Part model, mm, in its own coordinate system. A direction names the side the tool comes from. Round coordinates to 2 decimals unless told otherwise and drop trailing zeros. Write each loop counter-clockwise with the first axis right and the second up, starting at its lowest first coordinate (ties: lowest second). Pieces come first, ordered by that corner, then holes.
from build123d import *

# Parameters (mm, degrees)
F0_W     = 76.4351114631
F0_H     = 77.7774527669
F1_DEPTH = 50.8
F3_DEPTH = 77.7784527669
F4_R     = 7.4764365624
F5_DEPTH = 58.8116741145
F6_W     = 82.7689305879
F6_H     = 70.0802728534
F7_DEPTH = 12.7
F9_DEPTH = 90.4784527669


with BuildPart() as f1:
    # F0 (on Top) → F1 (new body)
    with BuildSketch(Plane.XY):
        with Locations((-38.2175557315, -38.8887263834)):
            Rectangle(F0_W, F0_H)
    extrude(amount=F1_DEPTH)

    # F2 (on face) → F3 (cut, through all)
    with BuildSketch(Plane.XZ.offset(77.7774527669)):
        Polygon((15.4465576634, -17.0485954732), (15.4465576634, 50.8), (-42.4766093493, 50.8), align=None)
    extrude(amount=-F3_DEPTH, mode=Mode.SUBTRACT)

    # F4 (on face) → F5 (cut, through all)
    with BuildSketch(Plane(origin=(0.5159375483, 0, 0.4404621285), x_dir=(0, 1, 0), z_dir=(0.760544385, 0, 0.6492859451))):
        with Locations((-41.5946096182, 34.9290184677)):
            Circle(F4_R)
    extrude(amount=-F5_DEPTH, mode=Mode.SUBTRACT)

    # F6 (on face) → F7 (join)
    with BuildSketch(Plane(origin=(0, 0, 0), x_dir=(-1, 0, 0), z_dir=(0, 1, 0))):
        with Locations((35.0506461691, 35.0401364267)):
            Rectangle(F6_W, F6_H)
    extrude(amount=F7_DEPTH)

    # F8 (on face) → F9 (cut, through all)
    with BuildSketch(Plane(origin=(0, 12.7, 0), x_dir=(-1, 0, 0), z_dir=(0, 1, 0))):
        Polygon((40.4624007642, 70.0802728534), (-6.3338191248, 70.0802728534), (-6.3338191248, 35.0401364267), align=None)
        Polygon((-6.3338191248, 0), (40.4624007642, 70.0802728534), (-6.3338191248, 35.0401364267), align=None)
    extrude(amount=-F9_DEPTH, mode=Mode.SUBTRACT)


solid = f1.part
Q1. Saw through at D-D, the plane y = 5. Write the cut outline in (x, z).
Q2. Saw through at C-C, the plane z = 63.5. Write the cut outline in (x, y), and give its area (3 significant figures).
Q3. Wall check: line 1 (Y direction, x = -35, z = 10.5); line 2 (Y direction, x = -27, z = 45); line 3 (Z direction, x = -41, y = -44.5). Give the ranges that are in metal, low to high.
Q4. Two-plate mould, pull along Y, no slides. Class faces 4 (the cylindrical face through (-41.6, -42.57, 20.16)), 5 (the flat face through (-16.737, 6.439, 34.55)), 6 (the flat face through (-38, 0, 48)), 7 (the flat face through (-44, 12.7, 28)): released by +Y, released by -Y, zero draft, split by the parting line, or undercut.
Q5. Drop flat-ended pins along their axis: P1, Ø12, axis at y = -11, z = 46, coming from the +X side; P2, Ø1, axis at x = -21.5, z = 38.5, coming from the -Y side; P3, Ø10, axis at x = -63, y = -57.5, coming from the +Z side; P4, Ø3, axis at x = -62, y = -28, coming from the -Z side. Give the stop position or say it passes through.
Q6. Saw through at A-A, the plane x = -70. Write the cut outline in (y, z), and give its area (3 significant figures).
Q7. Saw through at B-B, the plane y = -54. Write the cut outline in (x, z).
Q8. Tool access for faces 1 (the flat face through (-47, -77.777, 19)), 2 (the flat face through (-60, -38, 50.8)), 3 (the flat face through (-16.816, -39.433, 20.742)): list every direction of +Z, -Z, +X, -X, +Y, -Y with a clear straight run to the whole face (end or side of a thin tool).
Computed:
1. outline: (-76.44, 0) - (6.33, 0) - (-40.46, 70.08) - (-76.44, 70.08) - close
2. outline: (-76.44, 0) - (-36.07, 0) - (-36.07, 12.7) - (-76.44, 12.7) - close
2. area: 513 mm2
3. line 1: y = -77.78 to -47.77, -35.42 to 12.7
3. line 2: y = 0 to 12.7
3. line 3: z = 0 to 1.87, 19.98 to 49.07
4. face 4: undercut
4. face 5: zero draft
4. face 6: released by -Y
4. face 7: released by +Y
5. P1: stops at x = -33.26
5. P2: stops at y = 0
5. P3: stops at z = 50.8
5. P4: stops at z = 0
6. outline: (-77.78, 0) - (12.7, 0) - (12.7, 70.08) - (0, 70.08) - (0, 50.8) - (-77.78, 50.8) - close
6. area: 4,840 mm2
7. outline: (-76.44, 0) - (0, 0) - (0, 1.04) - (-42.48, 50.8) - (-76.44, 50.8) - close
8. face 1: +Z, -Z, +X, -X, -Y
8. face 2: +Z, +X, -X, -Y
8. face 3: +Z, +X, -Y
